Geometry: final body of the model. Coordinates: model frame, mm. A direction names the side the tool comes from. Round coordinates to 2 decimals unless told otherwise and drop trailing zeros. Order: outer loops, then holes, each group sorted by start corner. A loop starts at its lowest first (then second) coordinate and runs counter-clockwise, first axis right, second up. Notation, with made-up numbers: M -11,68.5 L 3,68.5 A22 ccw 3,93.5 Z; hole C 10.5,-20.75 d1. An arc over 180 degrees is marked long. Put each result on its own line as item: value. Start each with the question number.
1) Access query for faces 1 (the cylindrical face through (350, 105.6, 103.5)), 2 (the flat face through (395, 78, 104)). Directions: +Z, -Z, +X, -X, +Y, -Y. A direction counts if a zero-diameter tool reaches every point of the face in a straight line with its end or side. Return the directions, or none.
2) Section B-B, the plane x = 363.5. Return loops of the section in (y, z).
3) Section A-A, the plane y = 105.5. Return loops of the section in (x, z).
4) Section C-C, the plane z = 104.5. Return loops of the section in (x, y).
5) Material intervals for probe 1 along Y at (x, z) = (357.5, 101.75); probe 2 along Y at (x, z) = (353.5, 102), sorted ascending. Write a range as [from, to].
6) Draft query along Y for faces 3 (the flat face through (363, 110.5, 104)), 4 (the flat face through (367, 25, 104)), 5 (the flat face through (367, 77, 107)). Return one class per face: pulls with the +Y half, pulls with the -Y half, needs draft (parallel to the pull), parting line crosses it, or undercut.
from build123d import *

# Parameters (mm, degrees)
EXTRUDE_DEPTH = 7
BOX074_W      = 7
BOX074_H      = 105
BOX074_DEPTH  = 55


with BuildPart() as wirecut:
    # Sketch014 (on Face1 of Box074) → Extrude (new body)
    with BuildSketch(Plane(origin=(340, 25, 107), x_dir=(0, -1, 0), z_dir=(0, 0, 1))):
        with BuildLine():
            ThreePointArc((-75.5, 30), (-80.5, 35), (-85.5, 30))
            Line((-85.5, 30), (-85.5, 15))
            ThreePointArc((-85.5, 15), (-80.5, 10), (-75.5, 15))
            Line((-75.5, 30), (-75.5, 15))
        make_face()
    extrude(amount=-EXTRUDE_DEPTH)


with BuildPart() as cut003:
    # Box074 → Box074 (new body)
    with BuildSketch(Plane(origin=(340, 25, 107), x_dir=(0, 0, -1), z_dir=(1, 0, 0))):
        with Locations((3.5, 52.5)):
            Rectangle(BOX074_W, BOX074_H)
    extrude(amount=BOX074_DEPTH)

    # Cut003: cut Wirecut
    add(wirecut.part, mode=Mode.SUBTRACT)


solid = cut003.part
Result sheet:
1. face 1: +Z, -Z
1. face 2: +Z, -Z, +X, +Y, -Y
2. outline: M 25,100 L 100.5,100 L 100.5,107 L 25,107 Z; M 110.5,100 L 130,100 L 130,107 L 110.5,107 Z
3. outline: M 340,100 L 350,100 L 350,107 L 340,107 Z; M 375,100 L 395,100 L 395,107 L 375,107 Z
4. outline: M 340,25 L 395,25 L 395,130 L 340,130 Z; hole M 355,100.5 L 370,100.5 A5 ccw 370,110.5 L 355,110.5 A5 ccw Z
5. probe 1: y = [25, 100.5], [110.5, 130]
5. probe 2: y = [25, 100.73], [110.27, 130]
6. face 3: undercut
6. face 4: pulls with the -Y half
6. face 5: needs draft
